Geometry: final body of the model. Coordinates: model frame, mm. A direction names the side the tool comes from. Coordinates: 2 decimals unless noted, no trailing zeros. Write each loop counter-clockwise with the first axis right and the second up, starting at its lowest first coordinate (ties: lowest second). Pieces come first, ordered by that corner, then holes.
from build123d import *

# Parameters (mm, degrees)
SKETCH_1_R               = 1
SKETCH_1_W               = 16
SKETCH_1_H               = 9
SKETCH_1_W_2             = 7
SKETCH_1_H_2             = 7
EXTRUDE_1_DEPTH          = 3
SKETCH_2_W               = 7
SKETCH_2_H               = 2
EXTRUDE_2_DEPTH          = 10
CUT_EXTRUDE_1_DEPTH      = 35.150402633
CUT_EXTRUDE_1_DEPTH_BACK = 35.150402633
SKETCH_3_R               = 1.6
FILLET_1_R               = 2
SKETCH_4_W               = 1.2
SKETCH_4_H               = 3.5
CUT_EXTRUDE_3_DEPTH      = 10
EXTRUDE_3_DEPTH          = 7.5
EXTRUDE_6_DEPTH          = 5


with BuildPart() as part:
    # 草图1 → 凸台-拉伸1 (new body)
    with BuildSketch(Plane(origin=(0, 0, 0), x_dir=(1, 0, 0), z_dir=(0, 1, 0))):
        with BuildLine():
            Line((-10.5, -15), (10.5, -15))
            ThreePointArc((10.5, -15), (11.914213562, -14.414213562), (12.5, -13))
            Line((12.5, -13), (12.5, 13))
            ThreePointArc((12.5, 13), (11.914213562, 14.414213562), (10.5, 15))
            Line((10.5, 15), (-10.5, 15))
            ThreePointArc((-10.5, 15), (-11.914213562, 14.414213562), (-12.5, 13))
            Line((-12.5, 13), (-12.5, -13))
            ThreePointArc((-12.5, -13), (-11.914213562, -14.414213562), (-10.5, -15))
        make_face()
        with Locations(Location((-10, 7.5, 0), (0, 0, 270))):
            Circle(SKETCH_1_R, mode=Mode.SUBTRACT)
        with Locations(Location((10, 7.5, 0), (0, 0, 90))):
            Circle(SKETCH_1_R, mode=Mode.SUBTRACT)
        with Locations((0, 7.5)):
            Rectangle(SKETCH_1_W, SKETCH_1_H, mode=Mode.SUBTRACT)
        with Locations((6, -8.5)):
            Rectangle(SKETCH_1_W_2, SKETCH_1_H_2, mode=Mode.SUBTRACT)
        with Locations((-6, -8.5)):
            Rectangle(SKETCH_1_W_2, SKETCH_1_H_2, mode=Mode.SUBTRACT)
    extrude(amount=EXTRUDE_1_DEPTH)

    # 草图2 → 凸台-拉伸2 (add)
    with BuildSketch(Plane(origin=(0, 3, 0), x_dir=(1, 0, 0), z_dir=(0, 1, 0))):
        with Locations((-6, -4)):
            Rectangle(SKETCH_2_W, SKETCH_2_H)
        with Locations((-6, -13)):
            Rectangle(SKETCH_2_W, SKETCH_2_H)
        with Locations((6, -4)):
            Rectangle(SKETCH_2_W, SKETCH_2_H)
        with Locations((6, -13)):
            Rectangle(SKETCH_2_W, SKETCH_2_H)
    extrude(amount=EXTRUDE_2_DEPTH)

    # 草图3 → 切除-拉伸1 (cut, two sides: drawn at the far end of the back side and taken through both)
    with BuildSketch(Plane.XY.offset(14).offset(-CUT_EXTRUDE_1_DEPTH_BACK)):
        with Locations((-6, 11)):
            Circle(SKETCH_3_R)
        with Locations((-6, 5)):
            Circle(SKETCH_3_R)
        with Locations((6, 11)):
            Circle(SKETCH_3_R)
        with Locations((6, 5)):
            Circle(SKETCH_3_R)
    extrude(amount=CUT_EXTRUDE_1_DEPTH + CUT_EXTRUDE_1_DEPTH_BACK, mode=Mode.SUBTRACT)

    # 圆角1
    fillet_1_edges = [part.edges().sort_by_distance(p)[0] for p in [
        (2.5, 13, 4),
        (9.5, 13, 4),
        (2.5, 13, 13),
        (9.5, 13, 13),
        (-9.5, 13, 4),
        (-2.5, 13, 4),
        (-9.5, 13, 13),
        (-2.5, 13, 13),
    ]]
    fillet(fillet_1_edges, radius=FILLET_1_R)

    # 草图4 → 切除-拉伸3 (cut)
    with BuildSketch(Plane.XZ):
        with Locations((-8.6, -7.5)):
            Rectangle(SKETCH_4_W, SKETCH_4_H)
    extrude(amount=-CUT_EXTRUDE_3_DEPTH, mode=Mode.SUBTRACT)

    # 草图5 → 凸台-拉伸3 (add)
    with BuildSketch(Plane(origin=(0, 3, 0), x_dir=(1, 0, 0), z_dir=(0, 1, 0))):
        Polygon((-8, 3), (-8, 1), (10, 1), (10, 12), (8, 12), (8, 3), align=None)
    extrude(amount=EXTRUDE_3_DEPTH)

    # 草图8 → 凸台-拉伸6 (add)
    with BuildSketch(Plane(origin=(0, 10.5, 0), x_dir=(1, 0, 0), z_dir=(0, 1, 0))):
        Polygon((-8, 1), (-8, 2), (9, 2), (9, 12), (10, 12), (10, 1), align=None)
    extrude(amount=EXTRUDE_6_DEPTH)


solid = part.part
Item 1: Section D-D, the plane x = 4. Output: boundary loops of the cut face in (y, z), plus the area to 3 significant figures.
Derived:
outline: (0, -15) - (3, -15) - (3, -12) - (0, -12) - close; (0, -3) - (10.5, -3) - (10.5, -2) - (15.5, -2) - (15.5, -1) - (3, -1) - (3, 3) - (12.94, 3) - (12.94, 5) - (0, 5) - close; (0, 12) - (12.94, 12) - (12.94, 14) - (3, 14) - (3, 15) - (0, 15) - close
area: 102 mm2
Item 2: Set-up query: faces 5 (the cylindrical face through (-4.474, 11.481, 12.986)), 6 (the flat face through (-6, 8, 3)), 7 (the flat face through (9, 13, -7)), 8 (the flat face through (0, 1, -12)). Return all of +Z, -Z, +X, -X, +Y, -Y with unobstructed straight access to the full face (end or side cutting, diameter ignored); none if empty.
Derived:
face 5: +Z
face 6: +X, -X, +Y
face 7: -Z, -X, +Y
face 8: +Y, -Y
Item 3: Section B-B, the plane x = -10. Output: boundary loops of the cut face in (y, z).
Derived:
outline: (0, -15) - (3, -15) - (3, -8.5) - (0, -8.5) - close; (0, -6.5) - (3, -6.5) - (3, 15) - (0, 15) - close
Item 4: Pin query (flat end, axial travel): pin 1 (3.5 mm diameter, centred on x = -6, y = 11, fed in from -Z); pin 2 (2 mm diameter, centred on y = 11, z = 5, fed in from -X); pin 3 (2 mm diameter, centred on x = -2.5, y = 12.5, fed in from -Z). Return the tip coordinate at first contact, or that it passes through.
Derived:
pin 1: stops at z = -3
pin 2: stops at x = -9.5
pin 3: stops at z = -2
Item 5: Material intervals for probe 1 along Z at (x, y) = (3.75, 2.5); probe 2 along Y at (x, z) = (-6, 13.15); probe 3 along X at (y, z) = (5, 13.5), sorted ascending.
Derived:
probe 1: z = -15 to -12, -3 to 5, 12 to 15
probe 2: y = 0 to 3.4, 6.6 to 9.4, 12.6 to 13
probe 3: x = -9.5 to -7.6, -4.4 to -2.5, 2.5 to 4.4, 7.6 to 9.5
Item 6: Section C-C, the plane y = 1. Output: boundary loops of the cut face in (x, z), plus the area to 3 significant figures.
Derived:
outline: (-12.5, -13) arc R2 ccw to (-10.5, -15) - (10.5, -15) arc R2 ccw to (12.5, -13) - (12.5, 13) arc R2 ccw to (10.5, 15) - (-10.5, 15) arc R2 ccw to (-12.5, 13) - close; hole (-9.5, 5) - (-2.5, 5) - (-2.5, 12) - (-9.5, 12) - close; hole (-9.2, -9.25) - (-8, -9.25) - (-8, -12) - (8, -12) - (8, -3) - (-8, -3) - (-8, -5.75) - (-9.2, -5.75) - (-9.2, -6.9) arc R1 ccw (long way) to (-9.2, -8.1) - close; hole (2.5, 5) - (9.5, 5) - (9.5, 12) - (2.5, 12) - close; hole circle Ø2 at (10, -7.5)
area: 494 mm2
Item 7: Section A-A, the plane z = 11.5. Output: boundary loops of the cut face in (x, y).
Derived:
outline: (-12.5, 0) - (-9.5, 0) - (-9.5, 3) - (-12.5, 3) - close; (-2.5, 0) - (2.5, 0) - (2.5, 3) - (-2.5, 3) - close; (9.5, 0) - (12.5, 0) - (12.5, 3) - (9.5, 3) - close
Item 8: Pull-direction query (Y, two-part tool) for faces 1 (the cylindrical face through (7.526, 11.481, 3.986)), 2 (the cylindrical face through (-5.26, 3.58, 12.99)), 3 (the flat face through (6, 13, 4)), 4 (the flat face through (-8, 6, 5)); classes: released by +Y, released by -Y, zero draft, split by the parting line, or undercut.
Derived:
face 1: undercut
face 2: undercut
face 3: released by +Y
face 4: zero draft
